```python
from build123d import *

# Parameters (mm, degrees)
F1_DEPTH = 20
F2_W     = 20
F2_H     = 68
F3_DEPTH = 6.5
F4_W     = 20
F4_H     = 68
F5_DEPTH = 6.5


with BuildPart() as f1:
    # F0 (on Front) → F1 (new body)
    with BuildSketch(Plane.XZ):
        Polygon((-56.8088, 55.399762), (-56.8088, -12.600238), (-36.8088, -12.600238), (-36.8088, -24.600238), (119.704261, -24.600238), (119.704261, -12.600238), (139.704261, -12.600238), (139.704261, 55.399762), (119.704261, 55.399762), (119.704261, 67.399762), (-36.8088, 67.399762), (-36.8088, 55.399762), align=None)
    extrude(amount=F1_DEPTH)

    # F2 (on face) → F3 (cut)
    with BuildSketch(Plane.XZ.offset(20)):
        with Locations((129.704261, 21.399762)):
            Rectangle(F2_W, F2_H)
        with Locations((-46.8088, 21.399762)):
            Rectangle(F2_W, F2_H)
    extrude(amount=-F3_DEPTH, mode=Mode.SUBTRACT)

    # F4 (on face) → F5 (cut)
    with BuildSketch(Plane(origin=(0, 0, 0), x_dir=(-1, 0, 0), z_dir=(0, 1, 0))):
        with Locations((-129.704261, 21.399762)):
            Rectangle(F4_W, F4_H)
        with Locations((46.8088, 21.399762)):
            Rectangle(F4_W, F4_H)
    extrude(amount=-F5_DEPTH, mode=Mode.SUBTRACT)


solid = f1.part
```
CAD build for the part. Positions are in the model's coordinates, mm. A direction names the side the tool comes from. Round coordinates to 2 decimals unless told otherwise and drop trailing zeros. Order: outer loops, then holes, each group sorted by start corner. A loop starts at its lowest first (then second) coordinate and runs counter-clockwise, first axis right, second up.
Q1. Slice it at D-D (z = -15.5). Write the cut outline in (x, y).
Q2. Slice it at A-A (z = -1). Write the cut outline in (x, y), and give its area (3 significant figures).
Q3. Drop flat-ended pins along their axis: pin 1 (22 mm diameter, centred on x = 131.5, z = 18, fed in from +Y); pin 2 (22 mm diameter, centred on x = 133.5, z = 22.5, fed in from -Y); pin 3 (4 mm diameter, centred on y = -4, z = -13, fed in from +X). Give the stop position or say it passes through.
Q4. Slice it at C-C (x = -39.5). Write the cut outline in (y, z).
Q5. Which spindle directions (+Z, -Z, +X, -X, +Y, -Y) get a long thin tool onto all of the face, cutting with end or side? Do faces 1 (the flat face through (-47, -10, -12.6)), 2 (the flat face through (130, -10, -12.6)), 3 (the flat face through (-47, -10, 55.4)), 4 (the flat face through (130, -13.5, 22)), 5 (the flat face through (-47, -13.5, 22)). Say none if no direction does.
Q6. Wall check: L1, parallel to X at y = -6, z = -18.5; L2, parallel to Z at x = -48.5, y = -10.75. Give the ranges that are in metal, low to high.
Q7. Slice it at B-B (y = -11.5). Write the cut outline in (x, z), and give its area (3 significant figures).
Results below:
1. outline: (-36.81, -20) - (119.7, -20) - (119.7, 0) - (-36.81, 0) - close
2. outline: (-56.81, -13.5) - (-36.81, -13.5) - (-36.81, -20) - (119.7, -20) - (119.7, -13.5) - (139.7, -13.5) - (139.7, -6.5) - (119.7, -6.5) - (119.7, 0) - (-36.81, 0) - (-36.81, -6.5) - (-56.81, -6.5) - close
2. area: 3,410 mm2
3. pin 1: stops at y = -6.5
3. pin 2: stops at y = -13.5
3. pin 3: stops at x = 119.7
4. outline: (-13.5, -12.6) - (-6.5, -12.6) - (-6.5, 55.4) - (-13.5, 55.4) - close
5. face 1: -Z, -X, +Y, -Y
5. face 2: -Z, +X, +Y, -Y
5. face 3: +Z, -X, +Y, -Y
5. face 4: +Z, -Z, +X, -Y
5. face 5: +Z, -Z, -X, -Y
6. L1: x = -36.81 to 119.7
6. L2: z = -12.6 to 55.4
7. outline: (-56.81, -12.6) - (-36.81, -12.6) - (-36.81, -24.6) - (119.7, -24.6) - (119.7, -12.6) - (139.7, -12.6) - (139.7, 55.4) - (119.7, 55.4) - (119.7, 67.4) - (-36.81, 67.4) - (-36.81, 55.4) - (-56.81, 55.4) - close
7. area: 17,100 mm2
